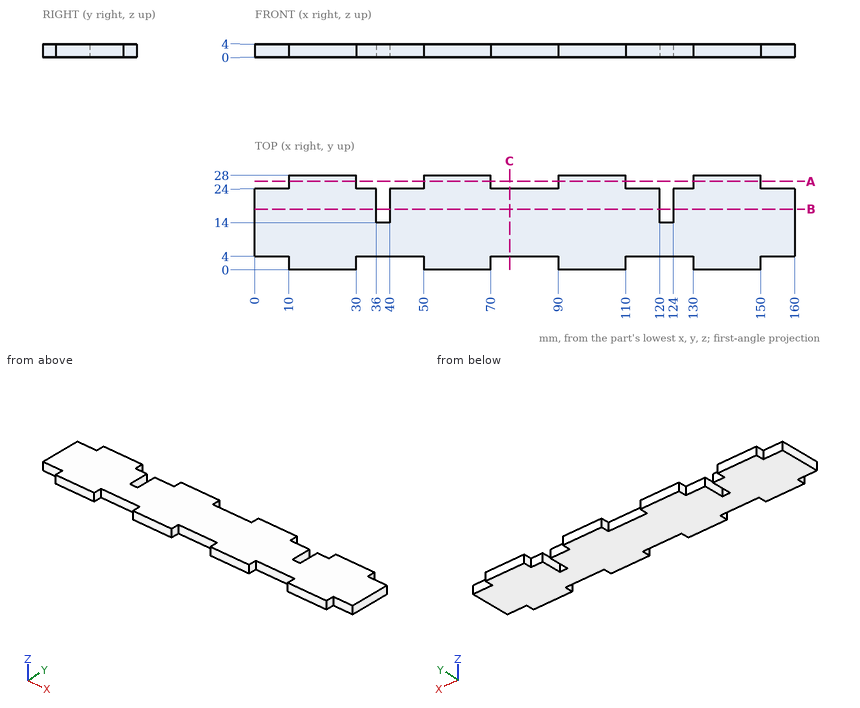
Print and shaded views of the part. All mm, measured from the part's lowest x, y and z. Round coordinates to 2 decimals unless told otherwise and drop trailing zeros. Order: outer loops, then holes, each group sorted by start corner. A loop starts at its lowest first (then second) coordinate and runs counter-clockwise, first axis right, second up. Notation, with made-up numbers: (-8.75, -35.5) - (18.25, -35.5) arc R6 ccw to (18.25, -25.5) - close; hole circle Ø7 at (10.5, 17.25). An arc over 180 degrees is marked (long way). Use a Markdown table: item, result.
1) Wall check: L1, parallel to X at y = 17.25, z = 2.35; L2, parallel to X at y = 2.5, z = 3.25; L3, parallel to Y at x = 83, z = 1.85. Give the ranges that are in metal, low to high.
Recorded:
| item | result |
|---|---|
| L1 | x = 0 to 36, 40 to 120, 124 to 160 |
| L2 | x = 10 to 30, 50 to 70, 90 to 110, 130 to 150 |
| L3 | y = 4 to 24 |
2) Saw through at C-C on x = 75.5. Write the cut outline in (y, z), and give its area (3 significant figures).
Recorded:
| item | result |
|---|---|
| outline | (4, 0) - (24, 0) - (24, 4) - (4, 4) - close |
| area | 80.0 mm² |
3) Flat gauge pins, fed straight in: pin 1 Ø2 at (y, z) = (25.5, 1) entering from +X; pin 2 Ø2 at (x, z) = (4, 2.5) entering from +Y; pin 3 Ø2 at (x, z) = (120, 2) entering from -Y. Where does each tip first touch, or does it go through?
Recorded:
| item | result |
|---|---|
| pin 1 | stops at x = 150 |
| pin 2 | stops at y = 24 |
| pin 3 | stops at y = 4 |
4) Saw through at A-A on y = 26.25. Write the cut outline in (x, z).
Recorded:
| item | result |
|---|---|
| outline | (10, 0) - (30, 0) - (30, 4) - (10, 4) - close; (50, 0) - (70, 0) - (70, 4) - (50, 4) - close; (90, 0) - (110, 0) - (110, 4) - (90, 4) - close; (130, 0) - (150, 0) - (150, 4) - (130, 4) - close |
5) Saw through at B-B on y = 18. Write the cut outline in (x, z), and give its area (3 significant figures).
Recorded:
| item | result |
|---|---|
| outline | (0, 0) - (36, 0) - (36, 4) - (0, 4) - close; (40, 0) - (120, 0) - (120, 4) - (40, 4) - close; (124, 0) - (160, 0) - (160, 4) - (124, 4) - close |
| area | 608 mm² |
